Autodesk Inventor part; units mm, degrees
ref_plane "작업 평면1" through (-420, 132.5, 170) normal (0, 0, 1) x (1, 0, 0)
ref_plane "YZ Plane" through (0, 0, 0) normal (1, 0, 0) x (0, 1, 0)
ref_plane "XZ Plane" through (0, 0, 0) normal (0, 1, 0) x (-1, 0, 0)
sketch "스케치1" plane through (0, 0, 0) normal (0, 1, 0) x (-1, 0, 0)
  line L0 (0, 475) -> (0, -475)
  line L1 (0, 475) -> (315, 475)
  line L2 (460, 170) -> (460, -170)
  line L3 (315, -475) -> (0, -475)
  line L4 (0, 0) -> (678.9617, 0) construction
  line L5 (460, 170) -> (995, 170)
  line L6 (995, -170) -> (460, -170)
  line L7 (460, 130) -> (995, 130)
  line L8 (995, -130) -> (460, -130)
  line L9 (995, 170) -> (995, 130)
  line L10 (995, -130) -> (995, -170)
  line L11 (0, 170) -> (-535, 170)
  line L12 (-535, -170) -> (0, -170)
  line L13 (-10, 130) -> (-535, 130)
  line L14 (-535, -130) -> (-10, -130)
  line L15 (-535, 170) -> (-535, 130)
  line L16 (-535, -130) -> (-535, -170)
  line L17 (460, 170) -> (460, 210)
  line L18 (460, -170) -> (460, -210)
  line L19 (460, 210) -> (315, 475)
  line L20 (460, -210) -> (315, -475)
  line L21 (420, 170) -> (420, 199.7721)
  line L22 (420, 199.7721) -> (291.2904, 435)
  line L23 (291.2904, 435) -> (40, 435)
  line L24 (40, 435) -> (40, -435)
  line L25 (40, -435) -> (291.2904, -435)
  line L26 (291.2904, -435) -> (420, -199.7721)
  line L27 (420, -199.7721) -> (420, 170)
  line L28 (460, -170) -> (0, -170)
  line L29 (-10, -130) -> (460, -130)
  line L30 (460, 130) -> (-10, 130)
  line L31 (460, 170) -> (0, 170)
  point P0 (460, 0)
  point P1 (995, -150)
  point P2 (-535, -150)
  point P3 (0, 130)
  point P4 (0, -130)
  point P5 (460, -190)
  point P6 (0, -130)
  point P7 (0, 130)
  dimension "d1" = 315
  dimension "d2" = 950
  dimension "d3" = 340
  dimension "d4" = 535
  dimension "d5" = 40
  dimension "d6" = 40
  dimension "d7" = 535
  dimension "d8" = 40
  dimension "d9" = 40
  dimension "d10" = 340
  dimension "d11" = 130
  dimension "d12" = 460
  dimension "d13" = 535
  dimension "d14" = 40
  dimension "d15" = 40
  dimension "d16" = 315
  dimension "d17" = 535
  dimension "d32" = 40
  dimension "d42" = 40
extrude "돌출1" add sketch "스케치1" along normal mid plane 265
sketch "스케치2" plane through (-995, 132.5, 170) normal (0, 0, 1) x (1, 0, 0)
  line L0 (535, -265) -> (535, 0)
  line L1 (0, 0) -> (535, 0)
  line L2 (0, -265) -> (0, 0)
  line L3 (535, -265) -> (0, -265)
  line L4 (1530, -265) -> (1530, 0)
  line L5 (995, 0) -> (1530, 0)
  line L6 (995, -265) -> (995, 0)
  line L7 (1530, -265) -> (995, -265)
  line L8 (500, -40) -> (500, -225)
  line L9 (535, -225) -> (0, -225)
  line L10 (40, -225) -> (40, -40)
  line L11 (40, -40) -> (535, -40)
  line L12 (1490, -40) -> (1490, -225)
  line L13 (1530, -225) -> (995, -225)
  line L14 (1035, -225) -> (1035, -40)
  line L15 (995, -40) -> (1490, -40)
  point P0 (995, -132.5)
  dimension "d20" = 40
  dimension "d21" = 40
  dimension "d30" = 185
  dimension "d31" = 40
extrude "돌출2" cut sketch "스케치2" against normal blind 8000 contours L9 L10 L11 L8 | L13 L14 L15 L12
extrude "돌출3" add sketch "스케치2" against normal blind 340 contours L3 L2 L9 L0 | L7 L6 L13 L4
sketch "스케치3" plane through (-955, -92.5, 170) normal (0, 1, 0) x (1, 0, 0)
  line L0 (70, 300) -> (70, 40)
  line L1 (1490, 300) -> (1380, 300)
  line L2 (1380, 300) -> (1380, 40)
  line L3 (1490, 0) -> (1490, 40)
  line L4 (1380, 40) -> (1490, 40)
  line L5 (70, 40) -> (-40, 40)
  line L6 (-40, 0) -> (-40, 340)
  line L7 (1490, 40) -> (1490, 300)
  line L8 (-40, 300) -> (0, 300)
  line L9 (-40, 300) -> (70, 300)
  point P0 (955, 170)
  dimension "d26" = 110
  dimension "d43" = 110
sketch "스케치4" plane through (0, 132.5, 0) normal (0, 1, 0) x (1, 0, 0)
  line L0 (0, -475) -> (0, -170)
  line L1 (0, -170) -> (535, -170)
  line L2 (535, -170) -> (535, -130)
  line L3 (535, -130) -> (0, -130)
  line L4 (0, 170) -> (0, 475)
  line L5 (0, 475) -> (-315, 475)
  line L6 (-315, 475) -> (-460, 210)
  line L7 (-460, 210) -> (-460, 170)
  line L8 (-460, 170) -> (-995, 170)
  line L9 (-995, 170) -> (-995, 130)
  line L10 (-995, 130) -> (-460, 130)
  line L11 (-460, 130) -> (-460, -130)
  line L12 (-460, -130) -> (-995, -130)
  line L13 (-995, -130) -> (-995, -170)
  line L14 (-995, -170) -> (-460, -170)
  line L15 (-460, -170) -> (-460, -210)
  line L16 (-460, -210) -> (-315, -475)
  line L17 (-315, -475) -> (0, -475)
  line L18 (-291.2904, -435) -> (-420, -199.7721)
  line L19 (-420, -199.7721) -> (-420, -170)
  line L20 (-420, -170) -> (-420, 130)
  line L21 (-420, 130) -> (-420, 199.7721)
  line L22 (-420, 199.7721) -> (-291.2904, 435)
  line L23 (-291.2904, 435) -> (-40, 435)
  line L24 (-40, 435) -> (-40, 170)
  line L25 (-40, 170) -> (-40, -130)
  line L26 (-40, -130) -> (-40, -435)
  line L27 (-40, -435) -> (-291.2904, -435)
  line L28 (-460, -170) -> (0, -170)
  line L29 (-460, -130) -> (0, -130)
  line L30 (-460, 170) -> (0, 170)
  line L31 (0, -130) -> (0, 130)
  line L32 (0, 130) -> (535, 130)
  line L33 (535, 130) -> (535, 170)
  line L34 (535, 170) -> (0, 170)
  line L35 (0, 130) -> (-460, 130)
  point P0 (0, 0)
  point P1 (-420, 170)
  point P2 (-420, -130)
  point P3 (-40, -170)
  point P4 (-420, -170)
  point P5 (-165.6452, 435)
  point P6 (-40, 130)
  point P7 (-420, 130)
  dimension "d33" = 40
  dimension "d46" = 40
  dimension "d47" = 90
  dimension "d48" = 265
sketch "스케치5" plane through (-460, 132.5, -130) normal (-1, 0, 0) x (0, 0, 1)
  line L0 (0, 0) -> (260, 0)
  line L1 (0, -225) -> (260, -225)
  line L2 (0, -40) -> (260, -40)
  line L3 (0, -225) -> (0, 0)
  line L4 (260, -225) -> (260, 0)
  point P0 (130, -132.5)
  point P1 (0, -265)
  point P2 (260, -265)
  dimension "d36" = 40
extrude "돌출6" cut sketch "스케치5" against normal blind 1000 contours L2 L4 L1 L3
ref_plane "작업 평면1" through (-420, 132.5, 170) normal (0, 0, 1) x (1, 0, 0)
sketch "스케치7" plane through (-420, 132.5, 170) normal (0, 0, 1) x (1, 0, 0)
  line L0 (0, 0) -> (380, 0)
  line L1 (0, -40) -> (390, -40)
  line L2 (0, 0) -> (380, 0)
  line L3 (0, 0) -> (0, -225)
  line L4 (0, -225) -> (380, -225)
  line L5 (380, 0) -> (380, -225)
  point P0 (420, -132.5)
  point P1 (380, -40)
  dimension "d39" = 40
extrude "돌출7" cut sketch "스케치7" against normal blind 350 contours L1 L5 L4 L3
extrude "돌출8" cut sketch "스케치3" against normal blind 265
extrude "돌출9" cut sketch "스케치4" against normal blind 225 contours L26 L27 L18 L19 L28 | L29 L20 L35 L25 | L30 L21 L22 L23 L24
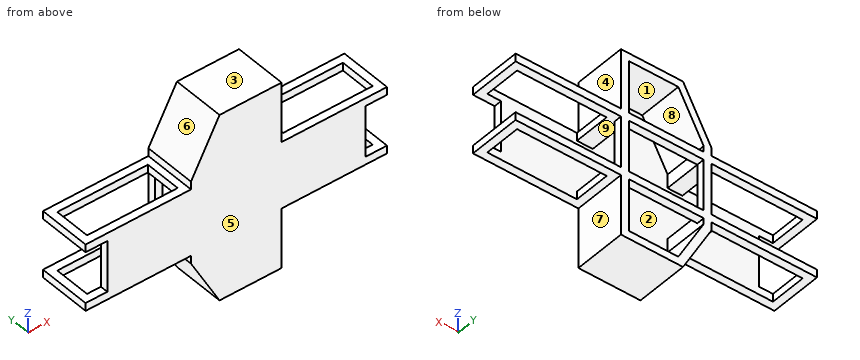
Geometry check sheet. Reference: the model listing, model coordinates, mm. Face numbers are marked on the shaded views. A direction names the side the tool comes from. Coordinates: 2 decimals unless noted, no trailing zeros. Order: outer loops, then holes, each group sorted by start corner. A loop starts at its lowest first (then second) coordinate and runs counter-clockwise, first axis right, second up. Notation, with made-up numbers: M 46.5,79.5 L 53.5,79.5 A29 ccw 53.5,117.5 Z; hole C 66,-27 d8. An arc over 180 degrees is marked long. Answer as a JSON object with one key per item and string values.
Q1. Tool access check on the marked faces 5, 6, 7, 8 and 9. Record the directions out of +Z, -Z, +X, -X, +Y, -Y that give a thin tool (end or side, any length) a straight path to the whole face; none if there is none.
Results are:
{"face 5": "+Z, -Z, +X, -X, -Y", "face 6": "+Z, -X, +Y, -Y", "face 7": "-Z, +X, +Y, -Y", "face 8": "+Y", "face 9": "+X"}
Q2. Scan lines: line 1 (Z direction, x = -485, y = -55.5); line 2 (Y direction, x = 130, z = -139.5); line 3 (X direction, y = 76, z = -145.5). Record each from-to range of solid material in increasing order.
Results are:
{"line 1": "z = -170 to -130, 130 to 170", "line 2": "y = -132.5 to -92.5, 92.5 to 132.5", "line 3": "x = -995 to -955, -495 to -420, -40 to 40, 495 to 535"}
Q3. Cross-section at A-A on z = 7. Record the cut outline in (x, y), and give its area (3 significant figures).
Results are:
{"outline": "M -885,-132.5 L 425,-132.5 L 425,-92.5 L -885,-92.5 Z; M -460,92.5 L -420,92.5 L -420,132.5 L -460,132.5 Z; M -40,92.5 L 0,92.5 L 0,132.5 L -40,132.5 Z", "area": "55,600 mm²"}
Q4. Cross-section at B-B on x = -846.5. Record the cut outline in (y, z), and give its area (3 significant figures).
Results are:
{"outline": "M -132.5,-170 L -92.5,-170 L -92.5,170 L -132.5,170 Z; M 92.5,-170 L 132.5,-170 L 132.5,-130 L 92.5,-130 Z; M 92.5,130 L 132.5,130 L 132.5,170 L 92.5,170 Z", "area": "16,800 mm²"}
Q5. Release check for a two-part mould opening along X. For the marked faces 1, 2, 3 and 4 record: released by +X, released by -X, zero draft, split by the parting line, or undercut.
Results are:
{"face 1": "undercut", "face 2": "undercut", "face 3": "zero draft", "face 4": "released by +X"}
Q6. Cross-section at C-C on y = -113. Record the cut outline in (x, z), and give its area (3 significant figures).
Results are:
{"outline": "M -995,-170 L -460,-170 L -460,-210 L -315,-475 L 0,-475 L 0,-170 L 535,-170 L 535,-130 L 425,-130 L 425,130 L 535,130 L 535,170 L 0,170 L 0,475 L -315,475 L -460,210 L -460,170 L -995,170 L -995,130 L -885,130 L -885,-130 L -995,-130 Z", "area": "705,000 mm²"}
Q7. Depth check by flat-ended pin: pin 1 Ø4 at (x, z) = (-377.5, -2.5) entering from +Y; pin 2 Ø6 at (y, z) = (-37, -311) entering from +X; pin 3 Ø6 at (y, z) = (-70.5, 321.5) entering from -X. Enter the tip coordinate at first touch or a pass-through.
Results are:
{"pin 1": "stops at y = -92.5", "pin 2": "stops at x = 0", "pin 3": "stops at x = -400.63"}
Q8. Cross-section at D-D on z = -241. Record the cut outline in (x, y).
Results are:
{"outline": "M -443.04,-132.5 L 0,-132.5 L 0,132.5 L -40,132.5 L -40,-92.5 L -397.44,-92.5 L -397.44,132.5 L -443.04,132.5 Z"}
